```python
from build123d import *

# Parameters (mm, degrees)
SKETCH1_W           = 330.2
SKETCH1_H           = 279.4
BOSS_EXTRUDE1_DEPTH = 6.35
SKETCH2_W           = 12.7
SKETCH2_H           = 152.4
CUT_EXTRUDE1_DEPTH  = 217.645770787
CAVITY1_START       = -5.196816792
CAVITY1_OUTLINE_R   = 12.7
CAVITY1_DEPTH       = 14.479849691


# Read off the part's stored shape, not the designer's step: Cavity1
with BuildPart() as part:
    # Sketch1 → Boss-Extrude1 (new, symmetric)
    with BuildSketch(Plane(origin=(0, 0, 0), x_dir=(1, 0, 0), z_dir=(0, 1, 0))):
        Rectangle(SKETCH1_W, SKETCH1_H)
    extrude(amount=BOSS_EXTRUDE1_DEPTH, both=True)

    # Sketch2 → Cut-Extrude1 (cut, through all)
    with BuildSketch(Plane(origin=(0, 6.35, 0), x_dir=(1, 0, 0), z_dir=(0, 1, 0))):
        with Locations((-107.95, 63.5)):
            Rectangle(SKETCH2_W, SKETCH2_H)
        with Locations((107.95, 63.5)):
            Rectangle(SKETCH2_W, SKETCH2_H)
    extrude(amount=-CUT_EXTRUDE1_DEPTH, mode=Mode.SUBTRACT)

    # Cavity1 outline → Cavity1 (cut)
    with BuildSketch(Plane(origin=(0, 0, 0), x_dir=(0.9999894493458413, 0.00458279136333027, 0.00031499257366167274), z_dir=(0.004593603922986451, -0.9976356448477001, -0.06857126900030612)).offset(CAVITY1_START)):
        with Locations((0.440476058, -29.695196787)):
            Circle(CAVITY1_OUTLINE_R)
    extrude(amount=CAVITY1_DEPTH, mode=Mode.SUBTRACT)


solid = part.part
```
Can you work these out from the model? Positions are in its coordinate system, mm. A direction names the side the tool comes from. Give positions to 0.01 mm unless a question says otherwise; leave off trailing zeros. Loops run counter-clockwise (first coordinate to the right, second up) from the corner with the lowest first, then second, coordinate; pieces in that order, holes last. Notation, with made-up numbers: M -38,71 L -30,71 A10 cw -30,84 Z; hole C -8,-39.75 d11. An arc over 180 degrees is marked long. One line per item, written item: value.
(1) Suppose I cut it at A-A on z = -122. List the corners of the cut face in (x, y) for me.
Returned:
outline: M -165.1,-6.35 L -114.3,-6.35 L -114.3,6.35 L -165.1,6.35 Z; M -101.6,-6.35 L 101.6,-6.35 L 101.6,6.35 L -101.6,6.35 Z; M 114.3,-6.35 L 165.1,-6.35 L 165.1,6.35 L 114.3,6.35 Z
(2) We'd pull the mould along X, two halves only. Please class faces 3 (the face through (-165.1, 0, 2)), 4 (the face through (-114.3, 0, -62)), 5 (the face through (139, 0, -139.7)), 6 (the face through (165.1, 0, 2)): released by +X, released by -X, zero draft, split by the parting line, or undercut.
Returned:
face 3: released by -X
face 4: undercut
face 5: zero draft
face 6: released by +X
(3) Which directions (+Z, -Z, +X, -X, +Y, -Y) give clear straight access to the entire face, cutting with the end or side of a thin tool? Please do faces 1 (the face through (-101.6, 0, -62)), 2 (the face through (-2, 0, 139.7)).
Returned:
face 1: -Z, +Y, -Y
face 2: +Z, +X, -X, +Y, -Y
(4) Will this pin go through, and if not, where does the flat tip stop? pin 1 (4 mm diameter, centred on x = 106, y = -0.5, fed in from -Z).
Returned:
pin 1: z = 12.7
(5) I need wall thicknesses on line 1 (X direction, y = 2.25, z = -93.5); line 2 (X direction, y = 0.25, z = -29); line 3 (X direction, y = -6, z = -40). Which ranges of each line are inside material? Lowest first, please.
Returned:
line 1: -165.1 to -114.3, -101.6 to 101.6, 114.3 to 165.1
line 2: -165.1 to -114.3, -101.6 to -12.23, 13.13 to 101.6, 114.3 to 165.1
line 3: -165.1 to -114.3, -101.6 to -7.6, 8.56 to 101.6, 114.3 to 165.1
